Part model, mm, in its own coordinate system. A direction names the side the tool comes from. Coordinates: 2 decimals unless noted, no trailing zeros. Write each loop counter-clockwise with the first axis right and the second up, starting at its lowest first coordinate (ties: lowest second). Pieces come first, ordered by that corner, then holes. Notation, with made-up numbers: M 28,16.5 L 68,16.5 A32 ccw 68,44.5 Z; hole C -27.75,-32 d10. An arc over 180 degrees is marked long. Use a Markdown table: item, result. Add a question column.
Q1. Pin check, flat tips, straight feed: pin 1 Ø5.5 at (x, z) = (-16.26, -16.26) entering from -Y; pin 2 Ø1.8 at (x, z) = (2.5, 21.5) entering from +Y. Stop position of each tip, or through.
Q2. Slice it at A-A on y = 59. Write the cut outline in (x, z), then the cut area to 3 significant figures.
Q3. Tool access for faces 1 (the cylindrical face through (-2.775, 33.507, -19.327)), 2 (the flat face through (-3, 41.479, 22)), 3 (the flat face through (-27, 13.369, 0)): list every direction of +Z, -Z, +X, -X, +Y, -Y with a clear straight run to the whole face (end or side of a thin tool).
Q4. Mould opens along Z. For faces 4 (the flat face through (-3, 13.479, 22)), 5 (the cylindrical face through (20.859, 30.566, 21.797)), 6 (the cylindrical face through (-25.136, 33.397, -0.233)), 7 (the cylindrical face through (-22.3, 1, 0)) say: released by +Z, released by -Z, zero draft, split by the parting line, or undercut.
Q5. Slice it at B-B on y = 51. Write the cut outline in (x, z).
Q6. Wall check: L1, parallel to X at y = 30.5, z = 18.5; L2, parallel to Z at x = 17.5, y = 21; L3, parallel to Z at x = 12, y = 55. Give the ranges that are in metal, low to high. Write a range as from..to.
from build123d import *

# Parameters (mm, degrees)
BOSS_EXTRUDE1_DEPTH     = 62
SKETCH2_R               = 18
BOSS_EXTRUDE2_DEPTH     = 2
SKETCH3_R               = 16
CUT_EXTRUDE1_DEPTH      = 74.545904033
CUT_EXTRUDE2_DEPTH      = 2
SKETCH5_R               = 3.5
CUT_EXTRUDE3_DEPTH      = 74.545904033
SKETCH7_W               = 48
SKETCH7_H               = 4
LPATTERN1_COUNT         = 9
LPATTERN1_PITCH         = 6
MIRROR1_COPY_1_SKETCH_W = 48
MIRROR1_COPY_1_SKETCH_H = 4
MIRROR1_COPY_2_SKETCH_W = 48
MIRROR1_COPY_2_SKETCH_H = 4
MIRROR1_COPY_3_SKETCH_W = 48
MIRROR1_COPY_3_SKETCH_H = 4
MIRROR1_COPY_4_SKETCH_W = 48
MIRROR1_COPY_4_SKETCH_H = 4
MIRROR1_COPY_5_SKETCH_W = 48
MIRROR1_COPY_5_SKETCH_H = 4
MIRROR1_COPY_6_SKETCH_W = 48
MIRROR1_COPY_6_SKETCH_H = 4
MIRROR1_COPY_7_SKETCH_W = 48
MIRROR1_COPY_7_SKETCH_H = 4
MIRROR1_COPY_8_SKETCH_W = 48
MIRROR1_COPY_8_SKETCH_H = 4
SKETCH10_W              = 48
SKETCH10_H              = 4
LPATTERN2_COUNT         = 9
LPATTERN2_PITCH         = 6


with BuildPart() as part:
    # Sketch1 → Boss-Extrude1 (new body)
    with BuildSketch(Plane(origin=(0, 0, 0), x_dir=(1, 0, 0), z_dir=(0, 1, 0))):
        with BuildLine():
            Line((-24, 22), (18, 22))
            ThreePointArc((18, 22), (20.828427125, 20.828427125), (22, 18))
            Line((22, 18), (22, -19))
            ThreePointArc((22, -19), (20.828427125, -21.828427125), (18, -23))
            Line((18, -23), (-24, -23))
            ThreePointArc((-24, -23), (-26.828427125, -21.828427125), (-28, -19))
            Line((-28, -19), (-28, 18))
            ThreePointArc((-28, 18), (-26.828427125, 20.828427125), (-24, 22))
        make_face()
    extrude(amount=BOSS_EXTRUDE1_DEPTH)

    # Sketch2 → Boss-Extrude2 (add)
    with BuildSketch(Plane(origin=(0, 62, 0), x_dir=(1, 0, 0), z_dir=(0, 1, 0))):
        with Locations(Location((0, 0, 0), (0, 0, 270))):
            Circle(SKETCH2_R)
    extrude(amount=BOSS_EXTRUDE2_DEPTH)

    # Sketch3 → Cut-Extrude1 (cut, through all)
    with BuildSketch(Plane(origin=(0, 64, 0), x_dir=(1, 0, 0), z_dir=(0, 1, 0))):
        with Locations(Location((0, 0, 0), (0, 0, 270))):
            Circle(SKETCH3_R)
    extrude(amount=-CUT_EXTRUDE1_DEPTH, mode=Mode.SUBTRACT)

    # Sketch4 → Cut-Extrude2 (cut)
    with BuildSketch(Plane.XZ):
        with BuildLine():
            Line((-20.306853537, -1.994120307), (-20.306853537, -2))
            Line((-20.306853537, -2), (-10.443807973, -2))
            Line((-10.443807973, -2), (-10.443807973, 2))
            Line((-10.443807973, 2), (-20.306853537, 2))
            Line((-20.306853537, 2), (-20.306853537, 1.994120307))
            ThreePointArc((-20.306853537, 1.994120307), (-22.300973844, 0), (-20.306853537, -1.994120307))
        make_face()
    extrude(amount=-CUT_EXTRUDE2_DEPTH, mode=Mode.SUBTRACT)

    # Sketch5 → Cut-Extrude3 (cut, through all)
    with BuildSketch(Plane.XZ):
        with Locations(Location((16.263455967, 16.263455967, 0), (0, 0, 270))):
            Circle(SKETCH5_R)
        with Locations(Location((16.263455967, -16.263455967, 0), (0, 0, 270))):
            Circle(SKETCH5_R)
        with Locations(Location((-16.263455967, -16.263455967, 0), (0, 0, 270))):
            Circle(SKETCH5_R)
        with Locations(Location((-16.263455967, 16.263455967, 0), (0, 0, 270))):
            Circle(SKETCH5_R)
    extrude(amount=-CUT_EXTRUDE3_DEPTH, mode=Mode.SUBTRACT)

    # Sketch7 → Cut-Revolve1 (revolve, cut)
    with BuildSketch(Plane(origin=(-3, 0, 0), x_dir=(0, 0, -1), z_dir=(1, 0, 0))):
        with Locations((43.326339521, 3.479284524)):
            Rectangle(SKETCH7_W, SKETCH7_H)
    cut_revolve1 = revolve(axis=Axis((-3, 5.479284524, -67.326339521), (0, -1, 0)), mode=Mode.SUBTRACT)

    # LPattern1: Cut-Revolve1 ×9
    with Locations(*[(0, i * LPATTERN1_PITCH, 0) for i in range(1, LPATTERN1_COUNT)]):
        add(cut_revolve1, mode=Mode.SUBTRACT)

    # Mirror1: Cut-Revolve1 across plane
    add(cut_revolve1.mirror(Plane.XY), mode=Mode.SUBTRACT)

    # Mirror1 copy 1 sketch → Mirror1 copy 1 (revolve, cut)
    with BuildSketch(Plane(origin=(-3, 6, 0), x_dir=(0, 0, 1), z_dir=(1, 0, 0))):
        with Locations((43.326339521, -3.479284524)):
            Rectangle(MIRROR1_COPY_1_SKETCH_W, MIRROR1_COPY_1_SKETCH_H)
    revolve(axis=Axis((-3, 11.479284524, 67.326339521), (0, 1, 0)), mode=Mode.SUBTRACT)

    # Mirror1 copy 2 sketch → Mirror1 copy 2 (revolve, cut)
    with BuildSketch(Plane(origin=(-3, 12, 0), x_dir=(0, 0, 1), z_dir=(1, 0, 0))):
        with Locations((43.326339521, -3.479284524)):
            Rectangle(MIRROR1_COPY_2_SKETCH_W, MIRROR1_COPY_2_SKETCH_H)
    revolve(axis=Axis((-3, 17.479284524, 67.326339521), (0, 1, 0)), mode=Mode.SUBTRACT)

    # Mirror1 copy 3 sketch → Mirror1 copy 3 (revolve, cut)
    with BuildSketch(Plane(origin=(-3, 18, 0), x_dir=(0, 0, 1), z_dir=(1, 0, 0))):
        with Locations((43.326339521, -3.479284524)):
            Rectangle(MIRROR1_COPY_3_SKETCH_W, MIRROR1_COPY_3_SKETCH_H)
    revolve(axis=Axis((-3, 23.479284524, 67.326339521), (0, 1, 0)), mode=Mode.SUBTRACT)

    # Mirror1 copy 4 sketch → Mirror1 copy 4 (revolve, cut)
    with BuildSketch(Plane(origin=(-3, 24, 0), x_dir=(0, 0, 1), z_dir=(1, 0, 0))):
        with Locations((43.326339521, -3.479284524)):
            Rectangle(MIRROR1_COPY_4_SKETCH_W, MIRROR1_COPY_4_SKETCH_H)
    revolve(axis=Axis((-3, 29.479284524, 67.326339521), (0, 1, 0)), mode=Mode.SUBTRACT)

    # Mirror1 copy 5 sketch → Mirror1 copy 5 (revolve, cut)
    with BuildSketch(Plane(origin=(-3, 30, 0), x_dir=(0, 0, 1), z_dir=(1, 0, 0))):
        with Locations((43.326339521, -3.479284524)):
            Rectangle(MIRROR1_COPY_5_SKETCH_W, MIRROR1_COPY_5_SKETCH_H)
    revolve(axis=Axis((-3, 35.479284524, 67.326339521), (0, 1, 0)), mode=Mode.SUBTRACT)

    # Mirror1 copy 6 sketch → Mirror1 copy 6 (revolve, cut)
    with BuildSketch(Plane(origin=(-3, 36, 0), x_dir=(0, 0, 1), z_dir=(1, 0, 0))):
        with Locations((43.326339521, -3.479284524)):
            Rectangle(MIRROR1_COPY_6_SKETCH_W, MIRROR1_COPY_6_SKETCH_H)
    revolve(axis=Axis((-3, 41.479284524, 67.326339521), (0, 1, 0)), mode=Mode.SUBTRACT)

    # Mirror1 copy 7 sketch → Mirror1 copy 7 (revolve, cut)
    with BuildSketch(Plane(origin=(-3, 42, 0), x_dir=(0, 0, 1), z_dir=(1, 0, 0))):
        with Locations((43.326339521, -3.479284524)):
            Rectangle(MIRROR1_COPY_7_SKETCH_W, MIRROR1_COPY_7_SKETCH_H)
    revolve(axis=Axis((-3, 47.479284524, 67.326339521), (0, 1, 0)), mode=Mode.SUBTRACT)

    # Mirror1 copy 8 sketch → Mirror1 copy 8 (revolve, cut)
    with BuildSketch(Plane(origin=(-3, 48, 0), x_dir=(0, 0, 1), z_dir=(1, 0, 0))):
        with Locations((43.326339521, -3.479284524)):
            Rectangle(MIRROR1_COPY_8_SKETCH_W, MIRROR1_COPY_8_SKETCH_H)
    revolve(axis=Axis((-3, 53.479284524, 67.326339521), (0, 1, 0)), mode=Mode.SUBTRACT)

    # Sketch10 → Cut-Revolve2 (revolve, cut)
    with BuildSketch(Plane.XY):
        with Locations((-49.135889072, 3.369439349)):
            Rectangle(SKETCH10_W, SKETCH10_H)
    cut_revolve2 = revolve(axis=Axis((-73.135889072, 5.369439349, 0), (0, -1, 0)), mode=Mode.SUBTRACT)

    # LPattern2: Cut-Revolve2 ×9
    with Locations(*[(0, i * LPATTERN2_PITCH, 0) for i in range(1, LPATTERN2_COUNT)]):
        add(cut_revolve2, mode=Mode.SUBTRACT)


solid = part.part
Recorded:
| question | item | result |
|---|---|---|
| 1 | pin 1 | through |
| 1 | pin 2 | y = 62 |
| 2 | outline | M -28,-18 A4 ccw -24,-22 L 18,-22 A4 ccw 22,-18 L 22,19 A4 ccw 18,23 L -24,23 A4 ccw -28,19 Z; hole C -16.26,-16.26 d7; hole C -16.26,16.26 d7; hole C 0,0 d32; hole C 16.26,-16.26 d7; hole C 16.26,16.26 d7 |
| 2 | area | 1,280 mm² |
| 3 | face 1 | -Z |
| 3 | face 2 | +Z |
| 3 | face 3 | -X |
| 4 | face 4 | zero draft |
| 4 | face 5 | released by +Z |
| 4 | face 6 | undercut |
| 4 | face 7 | undercut |
| 5 | outline | M -28,-18 A4 ccw -24,-22 L -18.8,-22 A48 cw 12.8,-22 L 18,-22 A4 ccw 22,-18 L 22,19 A4 ccw 18,23 L 15.42,23 A48 cw -21.42,23 L -24,23 A4 ccw -28,19 L -28,16.33 A48 cw -28,-16.33 Z; hole C -16.26,-16.26 d7; hole C -16.26,16.26 d7; hole C 0,0 d32; hole C 16.26,-16.26 d7; hole C 16.26,16.26 d7 |
| 6 | L1 | -28..-18.96, -13.57..13.57, 18.96..22 |
| 6 | L2 | -22..-19.54, -12.99..12.99, 19.54..23 |
| 6 | L3 | -22..-10.58, 10.58..23 |
